The listing builds one solid part. Answer for the finished solid, in the listing's coordinates (mm). A direction names the side the tool comes from. Coordinates: 2 decimals unless noted, no trailing zeros. Write each loop counter-clockwise with the first axis right and the second up, starting at its lowest first coordinate (ties: lowest second). Pieces come first, ordered by that corner, then holes. Notation, with made-up numbers: M 24.5,4.25 L 52.5,4.25 A28 cw 52.5,40.25 Z; hole C 23.25,45.25 d2. An arc over 180 degrees is marked long. Answer as a JSON object with one key per item and string values. Group by question number.
from build123d import *

# Parameters (mm, degrees)
BEAM_DEPTH        = 6.35
CENTER_R          = 25.4
CENTER1_DEPTH     = 6.35
RING_R            = 95.25
RING_R_2          = 92.075
RING1_DEPTH       = 6.35
CIRPATTERN3_COUNT = 4


with BuildPart() as part:
    # Beams → Beam (new body)
    with BuildSketch(Plane(origin=(0, 0, 0), x_dir=(1, 0, 0), z_dir=(0, 1, 0))):
        with BuildLine():
            Line((-91.855773498, 6.35), (-24.593444248, 6.35))
            ThreePointArc((-24.593444248, 6.35), (-25.4, 0), (-24.593444248, -6.35))
            Line((-24.593444248, -6.35), (-91.855773498, -6.35))
            ThreePointArc((-91.855773498, -6.35), (-92.075, 0), (-91.855773498, 6.35))
        make_face()
    beam = extrude(amount=BEAM_DEPTH)

    # Center → Center1 (add)
    with BuildSketch(Plane(origin=(0, 0, 0), x_dir=(1, 0, 0), z_dir=(0, 1, 0))):
        Circle(CENTER_R)
    extrude(amount=CENTER1_DEPTH)

    # Ring → Ring1 (add)
    with BuildSketch(Plane(origin=(0, 0, 0), x_dir=(1, 0, 0), z_dir=(0, 1, 0))):
        Circle(RING_R)
        Circle(RING_R_2, mode=Mode.SUBTRACT)
    extrude(amount=RING1_DEPTH)

    # CirPattern3: Beam ×4 about axis
    cirpattern3_axis = Axis((0, 0, 0), (0, 1, 0))
    for i in range(1, CIRPATTERN3_COUNT):
        add(beam.rotate(cirpattern3_axis, i * 360 / CIRPATTERN3_COUNT))


solid = part.part
Item 1: A cutting plane is placed at C-C, the plane z = -36.5. Write down the section's boundary in (x, y).
Item 2: A cutting plane is placed at A-A, the plane x = 31. Write down the section's boundary in (y, z), and give its area (3 significant figures).
Item 3: A cutting plane is placed at B-B, the plane y = 2.5. Write down the section's boundary in (x, z) (3 decimals).
Item 4: Consider L1, parallel to Z at x = 75, y = 1; L2, parallel to X at y = 4.5, z = -40.5; L3, parallel to Z at x = -40, y = 0.75. Determine where each line is inside the solid, lowest interval first. Write a range as from..to.
Item 5: A tool of negligible diameter and unlimited length cuts with its end or side. For faces 4 (the face through (6.35, 3, 58)), 5 (the face through (0, 0, 0)), from which of +Z, -Z, +X, -X, +Y, -Y can it reach the whole face along a straight path? Write none if from no direction.
Item 6: Flat-ended cylindrical pins translate along their axes: pin 1 Ø3 at (y, z) = (4, -71.5) entering from -X; pin 2 Ø3 at (y, z) = (1.5, 34) entering from +X; pin 3 Ø3 at (x, y) = (72, 3) entering from -Z; pin 4 Ø12 at (x, z) = (-26, 17.5) entering from -Y. Find the tip coordinate at first contact, or state that the pin passes through.
Item 7: For a pull along Z with two mould halves and no side action, classify faces 1 (the face through (-75.587, 3.131, 57.958)), 2 (the face through (0, 6.35, 0)), 3 (the face through (65.757, 3.131, -64.451)) as +Z half, -Z half, draft (parallel to the pull), parting line (faces both ways), or undercut.
Answer:
{
 "1": {"outline": "M -87.98,0 L -84.53,0 L -84.53,6.35 L -87.98,6.35 Z; M -6.35,0 L 6.35,0 L 6.35,6.35 L -6.35,6.35 Z; M 84.53,0 L 87.98,0 L 87.98,6.35 L 84.53,6.35 Z"},
 "2": {"outline": "M 0,-90.06 L 6.35,-90.06 L 6.35,-86.7 L 0,-86.7 Z; M 0,-6.35 L 6.35,-6.35 L 6.35,6.35 L 0,6.35 Z; M 0,86.7 L 6.35,86.7 L 6.35,90.06 L 0,90.06 Z", "area": "123 mm2"},
 "3": {"outline": "C 0,0 d190.5; hole M -91.856,-6.35 A92.075 ccw -6.35,-91.856 L -6.35,-24.593 A25.4 cw -24.593,-6.35 Z; hole M -91.856,6.35 L -24.593,6.35 A25.4 cw -6.35,24.593 L -6.35,91.856 A92.075 ccw Z; hole M 6.35,-91.856 A92.075 ccw 91.856,-6.35 L 24.593,-6.35 A25.4 cw 6.35,-24.593 Z; hole M 6.35,24.593 A25.4 cw 24.593,6.35 L 91.856,6.35 A92.075 ccw 6.35,91.856 Z"},
 "4": {"L1": "-58.72..-53.41, -6.35..6.35, 53.41..58.72", "L2": "-86.21..-82.69, -6.35..6.35, 82.69..86.21", "L3": "-86.44..-82.93, -6.35..6.35, 82.93..86.44"},
 "5": {"face 4": "+Y, -Y", "face 5": "+Z, -Z, +X, -X, -Y"},
 "6": {"pin 1": "x = -64.6", "pin 2": "x = 89.53", "pin 3": "z = -64.05", "pin 4": "y = 0"},
 "7": {"face 1": "parting line", "face 2": "draft", "face 3": "undercut"}
}
